Verification items for the finished model (mm, model axes). A direction names the side the tool comes from. Give positions to 0.01 mm unless a question says otherwise; leave off trailing zeros. Loops run counter-clockwise (first coordinate to the right, second up) from the corner with the lowest first, then second, coordinate; pieces in that order, holes last. Notation, with made-up numbers: (42.25, 56) - (86.25, 56) arc R20 ccw to (86.25, 62) - close; hole circle Ø7 at (59.5, -18). An arc over 180 degrees is marked (long way). One line per item, written item: value. Start each with the question number.
1. Sectioned sample at A-A (x = 0). Record the cut outline in (y, z), plus the area to 3 significant figures.
2. Scan lines: L1, parallel to X at y = 4, z = 56; L2, parallel to Z at x = 49.5, y = 1.25; L3, parallel to X at y = 1.25, z = 3. Record each from-to range of solid material in increasing order. Write a range as [from, to].
3. Mould release check, pull along Z, two halves, no side actions. Record for faces 3 (the flat face through (-7, 18, 85)), 4 (the cylindrical face through (97, 9, 0)), 5 (the cylindrical face through (-98.72, 9.13, 31.09)), 6 (the cylindrical face through (0, 9, -97)): pulls with the +Z half, pulls with the -Z half, needs draft (parallel to the pull), parting line crosses it, or undercut.
4. Access from +Z, -Z, +X, -X, +Y, -Y to the whole of each face (thin tool, end or side, straight path). Record for faces 1 (the flat face through (-68, 16, -43)), 2 (the cylindrical face through (-35.75, 7.888, -56.073)).
5. Sectioned sample at B-B (z = 0). Record the cut outline in (x, y).
6. Sectioned sample at D-D (z = -53). Record the cut outline in (x, y), plus the area to 3 significant figures.
7. Gauge pin test, flat ends, axial feed: pin 1 (1.5 mm diameter, centred on x = 71.5, y = 2, fed in from +Z); pin 2 (1 mm diameter, centred on x = 18, y = 11.5, fed in from -Z); pin 3 (1.5 mm diameter, centred on y = 2, z = -70.5, fed in from -X). Record the tip position at first contact, or that the pin passes through.
8. Sectioned sample at C-C (x = 33). Record the cut outline in (y, z).
Autodesk Inventor part; units mm, degrees
ref_plane "YZ Plane" through (0, 0, 0) normal (1, 0, 0) x (0, 1, 0)
ref_plane "XZ Plane" through (0, 0, 0) normal (0, 1, 0) x (-1, 0, 0)
ref_plane "XY Plane" through (0, 0, 0) normal (0, 0, 1) x (1, 0, 0)
sketch "Sketch1" plane through (0, 0, 0) normal (0, 0, 1) x (1, 0, 0)
  line L0 (-103.5, 0) -> (-103.5, 18)
  line L1 (-103.5, 18) -> (-83.5, 18)
  line L2 (-83.5, 18) -> (-83.5, 16)
  line L3 (-83.5, 16) -> (-80, 16)
  line L4 (-80, 16) -> (-80, 13.25)
  line L5 (-80, 13.25) -> (-76, 13.25)
  line L6 (-76, 13.25) -> (-76, 16)
  line L7 (-76, 16) -> (-66.5, 16)
  line L8 (-66.5, 16) -> (-66.5, 0)
  line L9 (-66.5, 0) -> (-103.5, 0)
  line L10 (0, -3.6) -> (0, 21.6)
  point P0 (0, 0)
  dimension "d0" = 103.5
  dimension "d1" = 20
  dimension "d2" = 4
  dimension "d3" = 76
  dimension "d4" = 66.5
  dimension "d5" = 18
  dimension "d6" = 2
  dimension "d7" = 2.75
revolve "Revolution1" add sketch "Sketch1" angle 360 about axis through (0, -10, 0) along (0, 1, 0)
sketch "Sketch2" plane through (0, 18, 0) normal (0, 1, 0) x (1, 0, 0)
  circle A0 centre (0, 0) radius 103.5
  point P0 (0, 91)
  dimension "d9" = 91
hole "Hole1" at (0, 18, -91) direction (0, -1, 0) diameter 12 end through all
pattern_circular "Circular Pattern1" count 8 over 360 about axis through (0, 8, 0) along (0, 1, 0) of "Hole1"
properties part number "CollarRingTop" material "Stainless Steel"
Results are:
1. outline: (0, -103.5) - (18, -103.5) - (18, -97) - (0, -97) - close; (0, -85) - (18, -85) - (18, -83.5) - (16, -83.5) - (16, -80) - (13.25, -80) - (13.25, -76) - (16, -76) - (16, -66.5) - (0, -66.5) - close; (0, 66.5) - (16, 66.5) - (16, 76) - (13.25, 76) - (13.25, 80) - (16, 80) - (16, 83.5) - (18, 83.5) - (18, 85) - (0, 85) - close; (0, 97) - (18, 97) - (18, 103.5) - (0, 103.5) - close
1. area: 810 mm^2
2. L1: x = [-87.04, -35.86], [35.86, 87.04]
2. L2: z = [-90.9, -44.41], [44.41, 90.9]
2. L3: x = [-103.46, -96.2], [-85.8, -66.43], [66.43, 85.8], [96.2, 103.46]
3. face 3: needs draft
3. face 4: undercut
3. face 5: parting line crosses it
3. face 6: undercut
4. face 1: +Y
4. face 2: +Y, -Y
5. outline: (-103.5, 0) - (-97, 0) - (-97, 18) - (-103.5, 18) - close; (-85, 0) - (-66.5, 0) - (-66.5, 16) - (-76, 16) - (-76, 13.25) - (-80, 13.25) - (-80, 16) - (-83.5, 16) - (-83.5, 18) - (-85, 18) - close; (66.5, 0) - (85, 0) - (85, 18) - (83.5, 18) - (83.5, 16) - (80, 16) - (80, 13.25) - (76, 13.25) - (76, 16) - (66.5, 16) - close; (97, 0) - (103.5, 0) - (103.5, 18) - (97, 18) - close
6. outline: (-88.9, 0) - (-40.17, 0) - (-40.17, 16) - (-54.47, 16) - (-54.47, 13.25) - (-59.92, 13.25) - (-59.92, 16) - (-64.52, 16) - (-64.52, 18) - (-88.9, 18) - close; (40.17, 0) - (88.9, 0) - (88.9, 18) - (64.52, 18) - (64.52, 16) - (59.92, 16) - (59.92, 13.25) - (54.47, 13.25) - (54.47, 16) - (40.17, 16) - close
6. area: 1,630 mm^2
7. pin 1: stops at z = 75.54
7. pin 2: stops at z = -102.01
7. pin 3: stops at x = -76.47
8. outline: (0, -98.1) - (18, -98.1) - (18, -76.7) - (16, -76.7) - (16, -72.88) - (13.25, -72.88) - (13.25, -68.46) - (16, -68.46) - (16, -57.73) - (0, -57.73) - close; (0, 57.73) - (16, 57.73) - (16, 68.46) - (13.25, 68.46) - (13.25, 72.88) - (16, 72.88) - (16, 76.7) - (18, 76.7) - (18, 98.1) - (0, 98.1) - close
